from build123d import *

# Parameters (mm, degrees)
F0_W     = 1070
F0_H     = 50
F1_DEPTH = 100
F2_T     = -4
F3_R     = 5
F5_D     = 22
F5_DEPTH = 4
F5_TIP   = 6.6094668093


with BuildPart() as f1:
    # F0 (on Front) → F1 (new body)
    with BuildSketch(Plane.XZ):
        Rectangle(F0_W, F0_H)
    extrude(amount=F1_DEPTH)

    # F2
    f2_openings = [f1.faces().sort_by_distance(p)[0] for p in [
        (-535, -50, 0),
        (535, -50, 0),
    ]]
    offset(amount=F2_T, openings=f2_openings)

    # F3
    f3_edges = [f1.edges().sort_by_distance(p)[0] for p in [
        (0, -96, -21),
        (0, -96, 21),
        (0, -4, -21),
        (0, -4, 21),
        (0, 0, 25),
        (0, 0, -25),
        (0, -100, 25),
        (0, -100, -25),
    ]]
    fillet(f3_edges, radius=F3_R)

    # F5
    with Locations(Plane.XZ.offset(100)):
        with Locations((0, 0)):
            Hole(F5_D / 2, depth=F5_DEPTH)
            with Locations((0, 0, -(F5_DEPTH + F5_TIP / 2))):  # 118° drill point
                Cone(0, F5_D / 2, F5_TIP, mode=Mode.SUBTRACT)


solid = f1.part
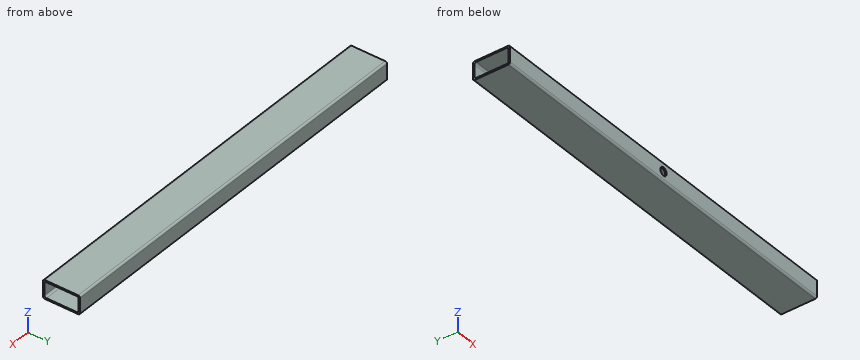
For this review, take the finished solid that the model builds, in its own axes (mm). Round coordinates to 2 decimals unless told otherwise and drop trailing zeros. Loops run counter-clockwise (first coordinate to the right, second up) from the corner with the lowest first, then second, coordinate; pieces in that order, holes last. Notation, with made-up numbers: (-14, 33.25) - (36, 33.25) arc R16 cw to (36, 61.25) - close; hole circle Ø5 at (-33, 5.25). An arc over 180 degrees is marked (long way). Answer as CSV lines item,"result".
(1) Insertion check: P1, Ø17.5, axis at x = 0, z = 0, coming from the -Y side. The pin has a flat end and moves straight along its axis. Give the tip position at first contact, or say it passes through.
Checked values:
P1,"stops at y = -4"
(2) Consider section B-B on z = 0. Give the boundary of the cut face in (x, y), then the cut area to 3 significant figures.
Checked values:
outline,"(-535, -100) - (-11, -100) - (-11, -96) - (-535, -96) - close; (-535, -4) - (535, -4) - (535, 0) - (-535, 0) - close; (11, -100) - (535, -100) - (535, -96) - (11, -96) - close"
area,"8,470 mm2"
(3) Consider section D-D on x = 0. Give the boundary of the cut face in (y, z), then the cut area to 3 significant figures.
Checked values:
outline,"(-100, -20) arc R5 ccw to (-95, -25) - (-5, -25) arc R5 ccw to (0, -20) - (0, 20) arc R5 ccw to (-5, 25) - (-95, 25) arc R5 ccw to (-100, 20) - (-100, 11) - (-96, 11) - (-96, 16) arc R5 cw to (-91, 21) - (-9, 21) arc R5 cw to (-4, 16) - (-4, -16) arc R5 cw to (-9, -21) - (-91, -21) arc R5 cw to (-96, -16) - (-96, -11) - (-100, -11) - close"
area,"1,050 mm2"
(4) Consider section A-A on y = -34.5. Give the boundary of the cut face in (x, z), then the cut area to 3 significant figures.
Checked values:
outline,"(-535, -25) - (535, -25) - (535, -21) - (-535, -21) - close; (-535, 21) - (535, 21) - (535, 25) - (-535, 25) - close"
area,"8,560 mm2"
(5) Consider section C-C on x = 155.5. Give the boundary of the cut face in (y, z).
Checked values:
outline,"(-100, -20) arc R5 ccw to (-95, -25) - (-5, -25) arc R5 ccw to (0, -20) - (0, 20) arc R5 ccw to (-5, 25) - (-95, 25) arc R5 ccw to (-100, 20) - close; hole (-96, -16) arc R5 ccw to (-91, -21) - (-9, -21) arc R5 ccw to (-4, -16) - (-4, 16) arc R5 ccw to (-9, 21) - (-91, 21) arc R5 ccw to (-96, 16) - close"
(6) Wall thickness on line 1 (Y direction, x = -460, z = 9); line 2 (Z direction, x = 396, y = -69); line 3 (X direction, y = -98.5, z = 0): over which ranges is each line inside the solid? List them lowest first.
Checked values:
line 1,"y = -100 to -96, -4 to 0"
line 2,"z = -25 to -21, 21 to 25"
line 3,"x = -535 to -11, 11 to 535"
